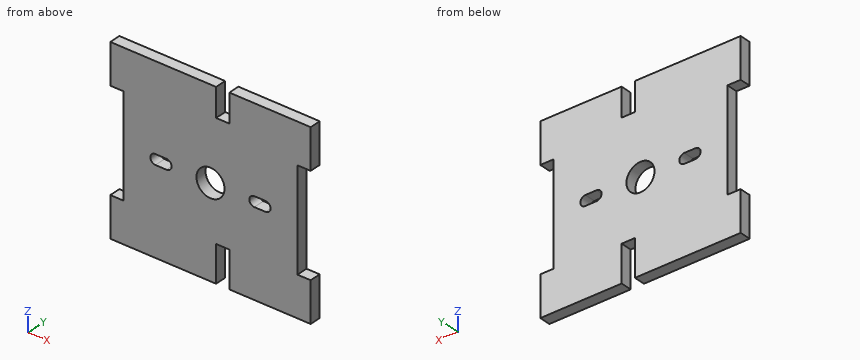
Autodesk Inventor part; units mm, degrees
ref_plane "YZ Plane" through (0, 0, 0) normal (1, 0, 0) x (0, 1, 0)
ref_plane "XZ Plane" through (0, 0, 0) normal (0, 1, 0) x (-1, 0, 0)
ref_plane "XY Plane" through (0, 0, 0) normal (0, 0, 1) x (1, 0, 0)
sketch "Sketch1" plane through (0, 0, 0) normal (0, 1, 0) x (-1, 0, 0)
  line L0 (-25, 22.5) -> (25, 22.5)
  line L1 (25, 22.5) -> (25, -22.5)
  line L2 (25, -22.5) -> (-25, -22.5)
  line L3 (-25, -22.5) -> (-25, 22.5)
  line L4 (-25, 22.5) -> (25, -22.5) construction
  line L5 (25, 22.5) -> (-25, -22.5) construction
  line L6 (25, -12.5) -> (21.7, -12.5)
  line L7 (21.7, -12.5) -> (21.7, 12.5)
  line L8 (21.7, 12.5) -> (25, 12.5)
  line L9 (25, 12.5) -> (25, -12.5)
  line L10 (-25, -12.5) -> (-21.7, -12.5)
  line L11 (-21.7, -12.5) -> (-21.7, 12.5)
  line L12 (-21.7, 12.5) -> (-25, 12.5)
  line L13 (-25, 12.5) -> (-25, -12.5)
  line L14 (-1.4, -22.5) -> (-4.7, -22.5)
  line L15 (-4.7, -22.5) -> (-4.7, -13.4)
  line L16 (-4.7, -13.4) -> (-1.4, -13.4)
  line L17 (-1.4, -13.4) -> (-1.4, -22.5)
  line L18 (-1.4, 22.5) -> (-4.7, 22.5)
  line L19 (-4.7, 22.5) -> (-4.7, 15.4)
  line L20 (-4.7, 15.4) -> (-1.4, 15.4)
  line L21 (-1.4, 15.4) -> (-1.4, 22.5)
  circle A0 centre (0, 0) radius 3.5
  line L22 (15, 0) -> (9.7, 0) construction
  line L23 (13.75, -1.25) -> (10.95, -1.25)
  line L24 (10.95, 1.25) -> (13.75, 1.25)
  arc A1 (13.75, -1.25) -> (13.75, 1.25) centre (13.75, 0) ccw
  arc A2 (10.95, 1.25) -> (10.95, -1.25) centre (10.95, 0) ccw
  line L25 (-9.7, 0) -> (-15, 0) construction
  line L26 (-10.95, -1.25) -> (-13.75, -1.25)
  line L27 (-13.75, 1.25) -> (-10.95, 1.25)
  arc A3 (-10.95, -1.25) -> (-10.95, 1.25) centre (-10.95, 0) ccw
  arc A4 (-13.75, 1.25) -> (-13.75, -1.25) centre (-13.75, 0) ccw
  line L28 (9.7, 0) -> (0, 0) construction
  line L29 (-9.7, 0) -> (0, 0) construction
  point P0 (21.7, 0)
  point P1 (12.35, 0)
  point P2 (-12.35, 0)
  dimension "d0" = 45
  dimension "d1" = 50
  dimension "d2" = 3.3
  dimension "d3" = 25
  dimension "d4" = 9.1
  dimension "d5" = 20.3
  dimension "d6" = 7
  dimension "d7" = 5.3
  dimension "d8" = 2.5
  dimension "d9" = 30
  dimension "d12" = 7.1
extrude "Extrusion1" add sketch "Sketch1" along normal blind 2.8 contours L0 L19 L20 L21 L1 L8 L7 L6 L2 L17 L16 L15 L3 L10 L11 L12
Can you work these out from the model? Positions are in its coordinate system, mm. Coordinates: 2 decimals unless noted, no trailing zeros. Loops run counter-clockwise (first coordinate to the right, second up) from the corner with the lowest first, then second, coordinate; pieces in that order, holes last.
1) Imagine slicing it at C-C on y = 1.1. State how many separate pieces and enclosed holes the cut face has, plus the area to 3 significant figures.
2) For pin 1 (1.4 mm diameter, centred on y = 1.5, z = 5.5, fed in from -X); pin 2 (0.8 mm diameter, centred on x = 3.5, y = 1, fed in from -Z), each with a flat end and sliding along its axis, tell me the tip position at first contact or that it passes through.
3) Imagine slicing it at B-B on z = 17. List the corners of the cut face in (x, y) for me.
4) I need wall thicknesses on probe 1 along X at (y, z) = (2.5, -17); probe 2 along Z at (x, y) = (-11, 2.35); probe 3 along Z at (x, y) = (0, 2.05). Which ranges of each line are inside material? Lowest first, please.
5) Imagine slicing it at A-A on x = -12.5. List the corners of the cut face in (y, z) for me.
Completed:
1. separate pieces: 1
1. enclosed holes: 3
1. area: 1,970 mm2
2. pin 1: stops at x = -21.7
2. pin 2: stops at z = -13.4
3. outline: (-25, 0) - (1.4, 0) - (1.4, 2.8) - (-25, 2.8) - close; (4.7, 0) - (25, 0) - (25, 2.8) - (4.7, 2.8) - close
4. probe 1: x = -25 to 1.4, 4.7 to 25
4. probe 2: z = -22.5 to -1.25, 1.25 to 22.5
4. probe 3: z = -22.5 to -3.5, 3.5 to 22.5
5. outline: (0, -22.5) - (2.8, -22.5) - (2.8, -1.25) - (0, -1.25) - close; (0, 1.25) - (2.8, 1.25) - (2.8, 22.5) - (0, 22.5) - close
